```python
from build123d import *

# Parameters (mm, degrees)
SKETCH1_R               = 5
BOSS_EXTRUDE1_DEPTH     = 5
SKETCH2_R               = 5.5
BOSS_EXTRUDE2_DEPTH     = 0.4
CUT_EXTRUDE1_DEPTH      = 6.4
SKETCH5_R               = 6
CUT_EXTRUDE2_DEPTH      = 6.5
CUT_EXTRUDE2_DEPTH_BACK = 6.5
CHAMFER4_SIZE           = 1
CHAMFER4_SIZE2          = 0.383864035


with BuildPart() as part:
    # Sketch1 → Boss-Extrude1 (new body)
    with BuildSketch(Plane(origin=(0, 0, 0), x_dir=(1, 0, 0), z_dir=(0, 1, 0))):
        Circle(SKETCH1_R)
    extrude(amount=BOSS_EXTRUDE1_DEPTH)

    # Sketch2 → Boss-Extrude2 (add)
    with BuildSketch(Plane(origin=(0, 5, 0), x_dir=(1, 0, 0), z_dir=(0, 1, 0))):
        Circle(SKETCH2_R)
    extrude(amount=BOSS_EXTRUDE2_DEPTH)

    # Sketch4 → Cut-Extrude1 (cut, through all)
    with BuildSketch(Plane(origin=(0, 5.4, 0), x_dir=(1, 0, 0), z_dir=(0, 1, 0))):
        with BuildLine():
            Line((2.295250379, 1.5), (2.295250379, -1.5))
            ThreePointArc((2.295250379, -1.5), (0, -3.795250379), (-2.295250379, -1.5))
            Line((-2.295250379, -1.5), (-2.295250379, 1.5))
            ThreePointArc((-2.295250379, 1.5), (0, 3.795250379), (2.295250379, 1.5))
        make_face()
    extrude(amount=-CUT_EXTRUDE1_DEPTH, mode=Mode.SUBTRACT)

    # Sketch5 → Cut-Extrude2 (cut, two sides)
    with BuildSketch(Plane(origin=(0, 0, 0), x_dir=(0, 0, -1), z_dir=(1, 0, 0))) as cut_extrude2_sk:
        with Locations((0, -1)):
            Circle(SKETCH5_R)
    extrude(amount=CUT_EXTRUDE2_DEPTH, mode=Mode.SUBTRACT)
    extrude(cut_extrude2_sk.sketch, amount=-CUT_EXTRUDE2_DEPTH_BACK, mode=Mode.SUBTRACT)

    # Chamfer4
    chamfer4_edges = [part.edges().sort_by_distance(p)[0] for p in [
        (0, 5.4, -3.795250379),
        (-2.295250379, 5.4, 0),
        (0, 5.4, 3.795250379),
        (2.295250379, 5.4, 0),
    ]]
    chamfer4_side = [part.faces().sort_by_distance(p)[0] for p in [
        (-5.344436508, 5.4, 0),
    ]]
    chamfer(chamfer4_edges, length=CHAMFER4_SIZE, length2=CHAMFER4_SIZE2, reference=chamfer4_side[0])


solid = part.part
```
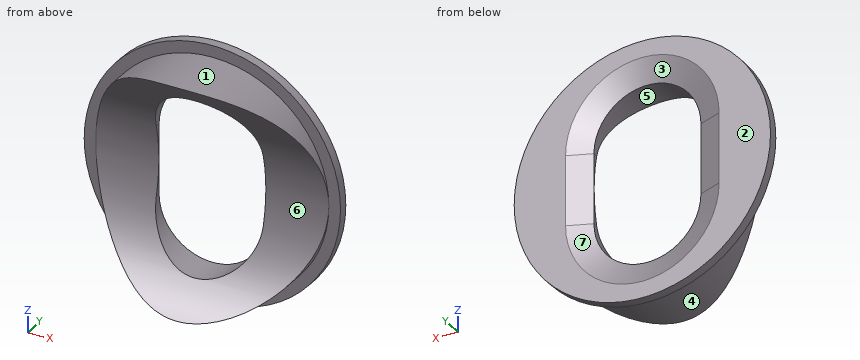
Input: part model. Units: mm. Frame: model coordinates. Face numbers are marked on the shaded views. A direction names the side the tool comes from. Round coordinates to 2 decimals unless told otherwise and drop trailing zeros. Loops run counter-clockwise (first coordinate to the right, second up) from the corner with the lowest first, then second, coordinate; pieces in that order, holes last. Notation, with made-up numbers: (58.25, 15.25) -> (106.25, 15.25) arc R19 ccw to (106.25, 24.25) -> close; hole circle Ø7 at (-38.5, -14). An arc over 180 degrees is marked (long way). Write each question's results on one line, items separated by ' | '.
1. First-contact query: P1, Ø4, axis at x = 0.5, z = -1, coming from the +Y side; P2, Ø4, axis at x = 0, z = 2.5, coming from the +Y side. Flat tips, straight axial feed; report the tip coordinate or a pass-through.
Geometry results:
P1: y = 5.09 | P2: y = 5.29
2. Ray query, line 1 (Z direction, x = 0, y = 4.2); line 2 (Z direction, x = 1.25, y = 4.05); line 3 (X direction, y = 4.55, z = -3.5). Return the intervals inside material, ascending. Write a range as from..to.
Geometry results:
line 1: -5..-3.8, 3.8..5 | line 2: -4.84..-3.43, 3.43..4.84 | line 3: -3.57..-1.13, 1.13..3.57
3. Set-up query: the marked faces 5, 6 and 7. Return all of +Z, -Z, +X, -X, +Y, -Y with unobstructed straight access to the full face (end or side cutting, diameter ignored); none if empty.
Geometry results:
face 5: +Y, -Y | face 6: +X, -X, -Y | face 7: +Y
4. Section C-C (x = 4.5). Return loops of the section in (y, z), and give its area (3 significant figures).
Geometry results:
outline: (4.59, -2.18) -> (5, -2.18) -> (5, -3.16) -> (5.4, -3.16) -> (5.4, 3.16) -> (5, 3.16) -> (5, 2.18) -> (4.59, 2.18) arc R6 cw to start | area: 3.12 mm2
5. Section D-D (y = 3.3). Return loops of the section in (x, z), and give its area (3 significant figures).
Geometry results:
outline: (-2.74, -4.18) arc R5 ccw to (2.74, -4.18) -> close; (-2.74, 4.18) -> (2.74, 4.18) arc R5 ccw to start | area: 6.06 mm2
6. Mould query, pull axis Z, two halves, no side actions, for the marked faces 1, 2, 3 and 4. Classes: +Z half, -Z half, draft (parallel to the pull), parting line (faces both ways), or undercut.
Geometry results:
face 1: +Z half | face 2: draft | face 3: undercut | face 4: -Z half
7. Section A-A (x = 0). Return loops of the section in (y, z).
Geometry results:
outline: (2.32, -5) -> (5, -5) -> (5, -5.5) -> (5.4, -5.5) -> (5.4, -4.8) -> (5.02, -3.8) -> (3.65, -3.8) arc R6 cw to start; (2.32, 5) arc R6 cw to (3.65, 3.8) -> (5.02, 3.8) -> (5.4, 4.8) -> (5.4, 5.5) -> (5, 5.5) -> (5, 5) -> close
8. Section B-B (y = 4). Return loops of the section in (x, z), and give its area (3 significant figures).
Geometry results:
outline: (-3.74, -3.32) arc R5 ccw to (3.74, -3.32) -> (1.4, -3.32) arc R2.3 cw to (-1.4, -3.32) -> close; (-3.74, 3.32) -> (-1.4, 3.32) arc R2.3 cw to (1.4, 3.32) -> (3.74, 3.32) arc R5 ccw to start | area: 15.6 mm2
